```python
from build123d import *

# Parameters (mm, degrees)
F0_W      = 63.5
F0_H      = 63.5
F1_DEPTH  = 63.5
F2_R      = 12.7
F3_R      = 3.2855032165
F4_DEPTH  = 10.16
F5_R      = 5.08
F6_DEPTH  = 2.54
F7_R      = 4.1642644098
F7_R_2    = 3.880802303
F8_DEPTH  = 10.16
F9_R      = 3.6538042468
F9_R_2    = 3.616555367
F9_R_3    = 3.5948118785
F9_R_4    = 3.6557525946
F9_R_5    = 3.6263948518
F10_DEPTH = 10.16
F11_R     = 3.6080090175
F11_R_2   = 3.6165563664
F11_R_3   = 3.6112952818
F12_DEPTH = 10.16
F13_R     = 3.6544564118
F13_R_2   = 3.6098297146
F13_R_3   = 3.6228239361
F13_R_4   = 3.6044825881
F14_DEPTH = 10.16


# Not quite as in the source:
# - a feature names something its author has since deleted; it is built from what else it names


with BuildPart() as f1:
    # F0 (on Top) → F1 (new body)
    with BuildSketch(Plane.XY):
        with Locations((-105.7584263082, 32.8302064445)):
            Rectangle(F0_W, F0_H)
    extrude(amount=F1_DEPTH)

    # F2
    f2_edges = [f1.edges().sort_by_distance(p)[0] for p in [
        (-74.008426, 32.830206, 0),
        (-137.508426, 32.830206, 0),
        (-105.758426, 1.080206, 0),
        (-137.508426, 1.080206, 31.75),
        (-74.008426, 1.080206, 31.75),
        (-137.508426, 32.830206, 63.5),
        (-105.758426, 64.580206, 0),
        (-137.508426, 64.580206, 31.75),
        (-105.758426, 64.580206, 63.5),
        (-74.008426, 64.580206, 31.75),
        (-74.008426, 32.830206, 63.5),
        (-105.758426, 1.080206, 63.5),
    ]]
    fillet(f2_edges, radius=F2_R)

    # F3 (on face) → F4 (cut)
    with BuildSketch(Plane.XY.offset(63.5)):
        with Locations((-105.7584263082, 32.8302064445)):
            Circle(F3_R)
    extrude(amount=-F4_DEPTH, mode=Mode.SUBTRACT)

    # F5 (on face) → F6 (cut)
    with BuildSketch(Plane(origin=(0, 0, 0), x_dir=(1, 0, 0), z_dir=(0, 0, -1))):
        with Locations((-111.8508055806, -21.4002064445)):
            Circle(F5_R)
        with Locations((-98.9837050438, -21.4002064445)):
            Circle(F5_R)
        with Locations((-111.8508055806, -32.8302064445)):
            Circle(F5_R)
        with Locations((-98.9837050438, -32.8302064445)):
            Circle(F5_R)
        with Locations((-111.8508055806, -44.2602064445)):
            Circle(F5_R)
        with Locations((-98.9837050438, -44.2602064445)):
            Circle(F5_R)
    extrude(amount=-F6_DEPTH, mode=Mode.SUBTRACT)

    # F7 (on face) → F8 (cut)
    with BuildSketch(Plane(origin=(-137.5084263082, 0, 0), x_dir=(0, -1, 0), z_dir=(-1, 0, 0))):
        with Locations((-40.1898002429, 39.1095937984)):
            Circle(F7_R)
        with Locations((-27.4898002429, 26.4095937984)):
            Circle(F7_R_2)
    extrude(amount=-F8_DEPTH, mode=Mode.SUBTRACT)

    # F9 (on face) → F10 (cut)
    with BuildSketch(Plane.YZ.offset(-74.0084263082)):
        with Locations((23.8499503234, 40.7302561211)):
            Circle(F9_R)
        with Locations((32.8302064445, 31.75)):
            Circle(F9_R_2)
        with Locations((41.8104625656, 40.7302561211)):
            Circle(F9_R_3)
        with Locations((23.8499503234, 22.7697438789)):
            Circle(F9_R_4)
        with Locations((41.8104625656, 22.7697438789)):
            Circle(F9_R_5)
    extrude(amount=-F10_DEPTH, mode=Mode.SUBTRACT)

    # F11 (on face) → F12 (cut)
    with BuildSketch(Plane(origin=(0, 64.5802064445, 0), x_dir=(-1, 0, 0), z_dir=(0, 1, 0))):
        with Locations((96.7781701871, 40.7302561211)):
            Circle(F11_R)
        with Locations((114.7386824292, 22.7697438789)):
            Circle(F11_R_2)
        with Locations((105.7584263082, 31.75)):
            Circle(F11_R_3)
    extrude(amount=-F12_DEPTH, mode=Mode.SUBTRACT)

    # F13 (on face) → F14 (cut)
    with BuildSketch(Plane.XZ.offset(-1.0802064445)):
        with Locations((-114.7386824292, 40.7302561211)):
            Circle(F13_R)
        with Locations((-96.7781701871, 40.7302561211)):
            Circle(F13_R_2)
        with Locations((-114.7386824292, 22.7697438789)):
            Circle(F13_R_3)
        with Locations((-96.7781701871, 22.7697438789)):
            Circle(F13_R_4)
    extrude(amount=-F14_DEPTH, mode=Mode.SUBTRACT)


solid = f1.part
```
Design review of the part built by this model. Coordinates are the model's own, in mm. A direction names the side the tool comes from. Round coordinates to 2 decimals unless told otherwise and drop trailing zeros. Write each loop counter-clockwise with the first axis right and the second up, starting at its lowest first coordinate (ties: lowest second). Pieces come first, ordered by that corner, then holes.
Item 1: Clearance check with flat-ended pins moving along their axes: pin 1 Ø6 at (y, z) = (25, 39.5) entering from +X; pin 2 Ø3 at (x, y) = (-97, 42.5) entering from -Z; pin 3 Ø2 at (y, z) = (22.5, 22) entering from +X; pin 4 Ø12 at (x, z) = (-80.5, 44.5) entering from +Y. State where each tip first meets the part, or that it passes through.
Item 2: We need section B-B on y = 51. Write out the cut boundary in (x, z), and give its area (3 significant figures).
Item 3: For faces 5 (the cylindrical face through (-103.097, 59.571, 34.191)), 6 (the flat face through (-106, 33, 53.34)), 7 (the cylindrical face through (-79.017, 23.374, 26.394)), 8 (the flat face through (-112, 33, 2.54)), 9 (the cylindrical face through (-100.385, 6.089, 40.889)), list the 3-axis set-ups (+Z, -Z, +X, -X, +Y, -Y) from which the entire face can be reached by the end or side of a thin tool; tool diameter is ignored.
Item 4: We need section A-A on z = 31.75. Write out the cut boundary in (x, y).
Item 5: We need section C-C on x = -120.5. Write out the cut boundary in (y, z), and give its area (3 significant figures).
Item 6: We need section D-D on x = -82. Write out the cut boundary in (y, z), and give its area (3 significant figures).
Item 7: For probe 1 along Z at (x, y) = (-125, 42); probe 2 along Y at (x, z) = (-95.5, 42); probe 3 along X at (y, z) = (25.5, 41), list the stretches that pass through material, from the lowest coordinate up.
Item 8: The part is to be moulded in two halves that separate along X. For faces 1 (the flat face through (-127.348, 40, 39)), 2 (the cylindrical face through (-107.16, 23.35, 1.25)), 3 (the flat face through (-106, 1.08, 31)), 4 (the cylindrical face through (-104.06, 32.61, 1.25)), say which applies: +X half, -X half, draft (parallel to the pull), parting line (faces both ways), or undercut.
Returned:
1. pin 1: stops at x = -74.01
1. pin 2: stops at z = 2.54
1. pin 3: stops at x = -84.17
1. pin 4: stops at y = 64.58
2. outline: (-137.51, 12.7) arc R12.7 ccw to (-124.81, 0) - (-86.71, 0) arc R12.7 ccw to (-74.01, 12.7) - (-74.01, 50.8) arc R12.7 ccw to (-86.71, 63.5) - (-124.81, 63.5) arc R12.7 ccw to (-137.51, 50.8) - close
2. area: 3,890 mm2
3. face 5: +Y
3. face 6: +Z
3. face 7: +X
3. face 8: -Z
3. face 9: -Y
4. outline: (-137.51, 13.78) arc R12.7 ccw to (-124.81, 1.08) - (-86.71, 1.08) arc R12.7 ccw to (-74.01, 13.78) - (-74.01, 29.21) - (-84.17, 29.21) - (-84.17, 36.45) - (-74.01, 36.45) - (-74.01, 51.88) arc R12.7 ccw to (-86.71, 64.58) - (-102.15, 64.58) - (-102.15, 54.42) - (-109.37, 54.42) - (-109.37, 64.58) - (-124.81, 64.58) arc R12.7 ccw to (-137.51, 51.88) - close
5. outline: (1.08, 12.7) arc R12.7 ccw to (13.78, 0) - (51.88, 0) arc R12.7 ccw to (64.58, 12.7) - (64.58, 50.8) arc R12.7 ccw to (51.88, 63.5) - (13.78, 63.5) arc R12.7 ccw to (1.08, 50.8) - close
5. area: 3,890 mm2
6. outline: (1.99, 12.7) arc R11.79 ccw to (13.78, 0.91) - (51.88, 0.91) arc R11.79 ccw to (63.68, 12.7) - (63.68, 50.8) arc R11.79 ccw to (51.88, 62.59) - (13.78, 62.59) arc R11.79 ccw to (1.99, 50.8) - close; hole circle Ø7.31 at (23.85, 22.77); hole circle Ø7.31 at (23.85, 40.73); hole circle Ø7.23 at (32.83, 31.75); hole circle Ø7.25 at (41.81, 22.77); hole circle Ø7.19 at (41.81, 40.73)
6. area: 3,480 mm2
7. probe 1: z = 0 to 63.5
7. probe 2: y = 11.24 to 54.42
7. probe 3: x = -137.51 to -84.17
8. face 1: -X half
8. face 2: undercut
8. face 3: draft
8. face 4: undercut
